Answer from the drawing. Dimensions are ordinates in mm from the lowest x, y and z of the part. Coordinates: 2 decimals unless noted, no trailing zeros. Write each loop counter-clockwise with the first axis right and the second up, starting at its lowest first coordinate (ties: lowest second). Pieces come first, ordered by that corner, then holes.
(1) Section C-C on x = 68 is taken. Write down the section's boundary in (y, z), then the cut area to 3 significant figures.
(2) Section B-B on z = 3.75 is taken. Write down the section's boundary in (x, y) (1 decimal).
(3) Section A-A on y = 190.5 is taken. Write down the section's boundary in (x, z), then the cut area to 3 significant figures.
(4) Find the intervals of material crossed by probe 1 along Y at (x, z) = (34, 11) (1 decimal); probe 2 along Y at (x, z) = (35.5, 7.25) (1 decimal); probe 3 along Y at (x, z) = (44.5, 7) (1 decimal), in increasing order.
(5) Given pin 1 (3 mm diameter, centred on x = 22.5, z = 10, fed in from -Y); pin 2 (1 mm diameter, centred on x = 61.5, z = 6, fed in from -Y) (1 decimal); pin 3 (6 mm diameter, centred on x = 37.5, z = 7, fed in from -Y); pin 4 (3 mm diameter, centred on x = 60.5, z = 3, fed in from -Y), each flat-ended and moving along its own axis, determine where each tip first touches the part or whether it passes through.
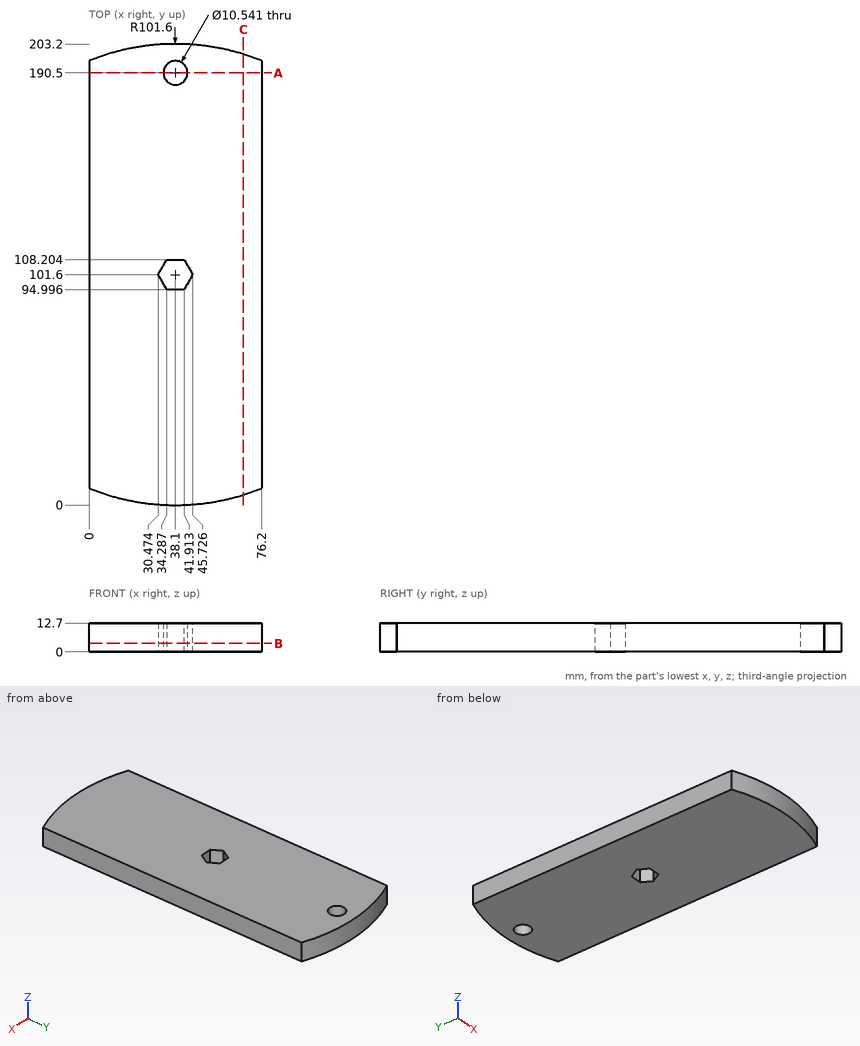
Response:
1. outline: (4.5, 0) - (198.7, 0) - (198.7, 12.7) - (4.5, 12.7) - close
1. area: 2,470 mm2
2. outline: (0, 7.4) arc R101.6 ccw to (76.2, 7.4) - (76.2, 195.8) arc R101.6 ccw to (0, 195.8) - close; hole (30.5, 101.6) - (34.3, 95) - (41.9, 95) - (45.7, 101.6) - (41.9, 108.2) - (34.3, 108.2) - close; hole circle Ø10.5 at (38.1, 190.5)
3. outline: (0, 0) - (32.83, 0) - (32.83, 12.7) - (0, 12.7) - close; (43.37, 0) - (76.2, 0) - (76.2, 12.7) - (43.37, 12.7) - close
3. area: 834 mm2
4. probe 1: y = 0.1 to 95.5, 107.7 to 187.2, 193.8 to 203.1
4. probe 2: y = 0 to 95, 108.2 to 185.9, 195.1 to 203.2
4. probe 3: y = 0.2 to 99.5, 103.7 to 203
5. pin 1: stops at y = 0.98
5. pin 2: stops at y = 2.6
5. pin 3: stops at y = 0
5. pin 4: stops at y = 2.17
